The listing builds one solid part. Answer for the finished solid, in the listing's coordinates (mm). A direction names the side the tool comes from. Give positions to 0.01 mm unless a question says otherwise; leave off trailing zeros. Write each loop counter-clockwise with the first axis right and the second up, starting at its lowest first coordinate (ties: lowest second). Pieces come first, ordered by that corner, then holes. Notation, with made-up numbers: (47, -20) - (68, -20) arc R8 ccw to (68, -15) - close; hole circle Ø7 at (23.5, 52). An arc over 180 degrees is marked (long way). Use a Markdown table: item, result. Add a question column.
from build123d import *

# Parameters (mm, degrees)
SKETCH1_W           = 9
SKETCH1_H           = 11
BOSS_EXTRUDE1_DEPTH = 15
CUT_EXTRUDE1_DEPTH  = 11
SKETCH3_R           = 3.15
CUT_EXTRUDE2_DEPTH  = 11
SKETCH4_W           = 2.979879399
SKETCH4_H           = 1.306685084
SKETCH4_W_2         = 2.979879398
SKETCH4_H_2         = 1.752870235
BOSS_EXTRUDE2_DEPTH = 4


with BuildPart() as part:
    # Sketch1 → Boss-Extrude1 (new body)
    with BuildSketch(Plane(origin=(0, 0, 0), x_dir=(1, 0, 0), z_dir=(0, 1, 0))):
        with Locations((0.651810585, 0.165738162)):
            Rectangle(SKETCH1_W, SKETCH1_H)
    extrude(amount=BOSS_EXTRUDE1_DEPTH)

    # Sketch2 → Cut-Extrude1 (cut)
    with BuildSketch(Plane(origin=(0, 15, 0), x_dir=(1, 0, 0), z_dir=(0, 1, 0))):
        with BuildLine():
            Line((-3.848189415, 2.350983054), (-6.541968857, 7.081862959))
            Line((-6.541968857, 7.081862959), (7.054694978, 6.829449645))
            Line((7.054694978, 6.829449645), (5.151810585, 2.350983054))
            ThreePointArc((5.151810585, 2.350983054), (0.651810585, 5.665738162), (-3.848189415, 2.350983054))
        make_face()
    extrude(amount=-CUT_EXTRUDE1_DEPTH, mode=Mode.SUBTRACT)

    # Sketch3 → Cut-Extrude2 (cut)
    with BuildSketch(Plane.XZ):
        with Locations((0.651810585, -0.165738162)):
            Circle(SKETCH3_R)
    extrude(amount=-CUT_EXTRUDE2_DEPTH, mode=Mode.SUBTRACT)

    # Sketch4 → Boss-Extrude2 (add)
    with BuildSketch(Plane.XY.offset(5.334261838)):
        with Locations((0.657536683, 14.037179674)):
            Rectangle(SKETCH4_W, SKETCH4_H)
        with Locations((0.588068697, 8.251967659)):
            Rectangle(SKETCH4_W_2, SKETCH4_H_2)
    extrude(amount=BOSS_EXTRUDE2_DEPTH)


solid = part.part
1. The part is cut by section D-D (z = -2.75). Give the vertices of the cut face in (x, y), and give its area (3 significant figures).
2. Consider L1, parallel to Y at x = -1.5, z = 0.75; L2, parallel to Z at x = 2, y = 9.5; L3, parallel to X at y = 7.25, z = 0.5. Determine where each line is inside the solid, lowest interval first. Write a range as [from, to].
3. Given P1, Ø1.5, axis at x = 0.5, z = 8.5, coming from the +Y side; P2, Ø1.5, axis at x = 1.5, z = 6.5, coming from the -Y side; P3, Ø1.4, axis at y = 8, z = 8, coming from the -X side, each flat-ended and moving along its own axis, determine where each tip first touches the part or whether it passes through.
4. Which of the six approach directions +Z, -Z, +X, -X, +Y, -Y give full straight-line access (tool end or side, diameter ignored) to faces 4 (the flat face through (1, 14.691, 7)), 5 (the flat face through (2.147, 14, 7)), 6 (the flat face through (1, 13.384, 7))?
5. The part is cut by section A-A (z = 7). Give the vertices of the cut face in (x, y), and give its area (3 significant figures).
6. For a pull along X with two mould halves and no side action, classify faces 1 (the cylindrical face through (-0.03, 5.42, -3.24)), 2 (the flat face through (-3.848, 7, 1)), 3 (the flat face through (1, 9.128, 7)) as released by +X, released by -X, zero draft, split by the parting line, or undercut.
7. The part is cut by section B-B (y = 8). Give the vertices of the cut face in (x, z), and give its area (3 significant figures).
8. The part is cut by section C-C (x = -1.25). Give the vertices of the cut face in (y, z), and give its area (3 significant figures).
Check values:
| question | item | result |
|---|---|---|
| 1 | outline | (-3.85, 0) - (-1.15, 0) - (-1.15, 11) - (2.45, 11) - (2.45, 0) - (5.15, 0) - (5.15, 4) - (5.01, 4) - (5.01, 15) - (-3.7, 15) - (-3.7, 4) - (-3.85, 4) - close |
| 1 | area | 92.2 mm2 |
| 2 | L1 | y = [11, 15] |
| 2 | L2 | z = [-5.47, -3.01], [2.68, 5.33] |
| 2 | L3 | x = [-3.85, -2.43], [3.73, 5.15] |
| 3 | P1 | stops at y = 14.69 |
| 3 | P2 | stops at y = 7.38 |
| 3 | P3 | stops at x = -0.9 |
| 4 | face 4 | +Z, +X, -X, +Y |
| 4 | face 5 | +Z, +X, +Y, -Y |
| 4 | face 6 | +Z, +X, -X |
| 5 | outline | (-0.9, 7.38) - (2.08, 7.38) - (2.08, 9.13) - (-0.9, 9.13) - close; (-0.83, 13.38) - (2.15, 13.38) - (2.15, 14.69) - (-0.83, 14.69) - close |
| 5 | area | 9.12 mm2 |
| 6 | face 1 | undercut |
| 6 | face 2 | released by -X |
| 6 | face 3 | zero draft |
| 7 | outline | (-3.85, -2.35) arc R4.71 ccw to (5.15, -2.35) - (5.15, 5.33) - (2.08, 5.33) - (2.08, 9.33) - (-0.9, 9.33) - (-0.9, 5.33) - (-3.85, 5.33) - close; hole circle Ø6.3 at (0.65, -0.17) |
| 7 | area | 71.8 mm2 |
| 8 | outline | (0, -5.67) - (4, -5.67) - (4, -5.26) - (15, -5.26) - (15, 5.33) - (0, 5.33) - (0, 2.35) - (11, 2.35) - (11, -2.68) - (0, -2.68) - close |
| 8 | area | 105 mm2 |
